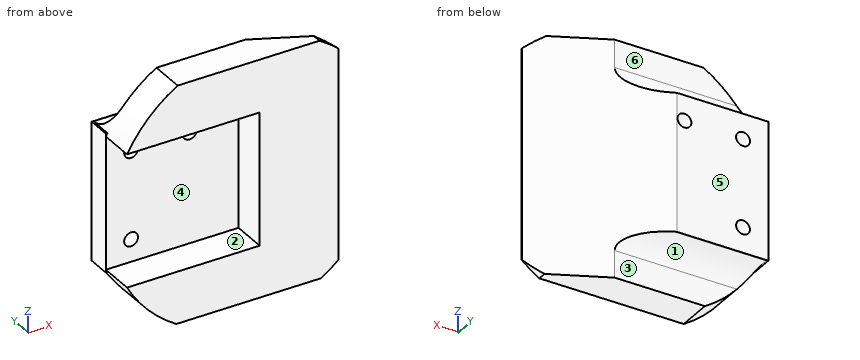
from build123d import *

# Parameters (mm, degrees)
PAD009_DEPTH    = 3
SKETCH023_W     = 15
SKETCH023_H     = 12
SKETCH023_R     = 0.6
PAD010_DEPTH    = 2
POCKET009_DEPTH = 20.546094
FILLET002_R     = 1.9


with BuildPart() as part:
    # Sketch024 → Pad009 (new body)
    with BuildSketch(Plane.XZ):
        with BuildLine():
            Line((-23.5, 5.75), (-12, 5.75))
            Line((-12, 5.75), (-12, -5.75))
            Line((-12, -5.75), (-23.5, -5.75))
            ThreePointArc((-23.5, -5.75), (-21.658628, -8.274119), (-19.228067, -10.237331))
            Line((-19.228067, -10.237331), (-6.706558, -10.237331))
            ThreePointArc((-6.706558, -10.237331), (-5.923041, -9.714846), (-5.182908, -9.132527))
            Line((-5.182908, 9.132527), (-5.182908, -9.132527))
            ThreePointArc((-5.182908, 9.132527), (-5.978311, 9.754684), (-6.823207, 10.307762))
            Line((-19.111419, 10.307762), (-6.823207, 10.307762))
            ThreePointArc((-19.111419, 10.307762), (-21.611511, 8.323331), (-23.5, 5.75))
        make_face()
    extrude(amount=-PAD009_DEPTH)

    # Sketch023 (on Face12 of Pad009) → Pad010 (join)
    with BuildSketch(Plane(origin=(0, 3, 0), x_dir=(1, 0, 0), z_dir=(0, 1, 0))):
        with Locations((-16, 0)):
            Rectangle(SKETCH023_W, SKETCH023_H)
        with Locations((-21.31, -3.81)):
            Circle(SKETCH023_R, mode=Mode.SUBTRACT)
        with Locations((-21.31, 3.81)):
            Circle(SKETCH023_R, mode=Mode.SUBTRACT)
        with Locations((-16.23, -3.81)):
            Circle(SKETCH023_R, mode=Mode.SUBTRACT)
    extrude(amount=PAD010_DEPTH)

    # Sketch026 (on Face2 of Pad010) → Pocket009 (cut, through all)
    with BuildSketch(Plane(origin=(0, 0, 10.307762), x_dir=(-1, 0, 0), z_dir=(0, 0, 1))):
        Polygon((5.151306, 0), (15.6, -5.012868), (5.151306, -5.012868), align=None)
    extrude(amount=-POCKET009_DEPTH, mode=Mode.SUBTRACT)

    # Fillet002
    fillet002_edges = [part.edges().sort_by_distance(p)[0] for p in [
        (-17.382023, 3, 6),
        (-17.382023, 3, -6),
    ]]
    fillet(fillet002_edges, radius=FILLET002_R)


with BuildPart() as part_1:
    # Body003 placement: moved
    add(part.part.moved(Location((0, 0.6, 0))))


solid = part_1.part
Could you check a few things on this model? Use its own coordinates, in mm. Face numbers are marked on the shaded views. A direction names the side the tool comes from. Coordinates: 2 decimals unless noted, no trailing zeros. Loops run counter-clockwise (first coordinate to the right, second up) from the corner with the lowest first, then second, coordinate; pieces in that order, holes last.
1. For P1, Ø1.4, axis at x = -16.23, z = 3.81, coming from the -Y side; P2, Ø1.5, axis at y = 2, z = -2, coming from the -X side; P3, Ø1.2, axis at x = -16, z = 8.5, coming from the +Y side, each with a flat end and sliding along its axis, tell me the tip position at first contact or that it passes through.
2. Imagine slicing it at D-D (y = 3.95). Please give me the cut outline in (x, z).
3. We'd pull the mould along Z, two halves only. Please class the marked faces 1, 2 and 3: released by +Z, released by -Z, zero draft, split by the parting line, or undercut.
4. I need wall thicknesses on L1, parallel to Z at x = -21.31, y = 4.6; L2, parallel to Z at x = -21.31, y = 4.2; L3, parallel to X at y = 4.6, z = 3.81. Which ranges of each line are inside material? Lowest first, please.
5. Imagine slicing it at B-B (x = -16.23). Please give me the cut outline in (y, z), and give its area (3 significant figures).
6. Imagine slicing it at C-C (z = 3.81). Give the number of separate pieces and of enclosed holes in the cut face, and give its area (3 significant figures).
7. For the marked faces 4, 5 and 6, which set-ups out of +Z, -Z, +X, -X, +Y, -Y let a thin tool reach every point of the face, with its end or its side?
Computed values:
1. P1: stops at y = 3.6
1. P2: stops at x = -12
1. P3: stops at y = 3.6
2. outline: (-23.5, -6) - (-23.36, -6) arc R12 ccw to (-22.85, -6.8) - (-12.13, -6.8) - (-12.13, 6.8) - (-22.85, 6.8) arc R12 ccw to (-23.36, 6) - (-23.5, 6) - close; hole circle Ø1.2 at (-21.31, -3.81); hole circle Ø1.2 at (-21.31, 3.81); hole circle Ø1.2 at (-16.23, 3.81)
3. face 1: released by -Z
3. face 2: undercut
3. face 3: zero draft
4. L1: z = -6.23 to -4.41, -3.21 to 3.21, 4.41 to 6.23
4. L2: z = -6.51 to -4.41, -3.21 to 3.21, 4.41 to 6.51
4. L3: x = -23.5 to -21.91, -20.71 to -16.83, -15.63 to -13.49
5. outline: (0.6, -10.24) - (3.6, -10.24) - (3.6, -7.9) arc R1.9 cw to (5.5, -6) - (5.6, -6) - (5.6, 3.21) - (3.6, 3.21) - (3.6, -5.75) - (0.6, -5.75) - close; (0.6, 5.75) - (3.6, 5.75) - (3.6, 4.41) - (5.6, 4.41) - (5.6, 6) - (5.5, 6) arc R1.9 cw to (3.6, 7.9) - (3.6, 10.31) - (0.6, 10.31) - close
5. area: 50.3 mm2
6. separate pieces: 3
6. enclosed holes: 0
6. area: 26.4 mm2
7. face 4: -X, -Y
7. face 5: +Z, -Z, +X, -X, +Y
7. face 6: +Z, +X, -X, +Y
